Source: CAD feature listing. Evaluate the final solid. Frame: model axes, mm. Face numbers are marked on the shaded views. A direction names the side the tool comes from. Give positions to 0.01 mm unless a question says otherwise; leave off trailing zeros. Order: outer loops, then holes, each group sorted by start corner. A loop starts at its lowest first (then second) coordinate and runs counter-clockwise, first axis right, second up.
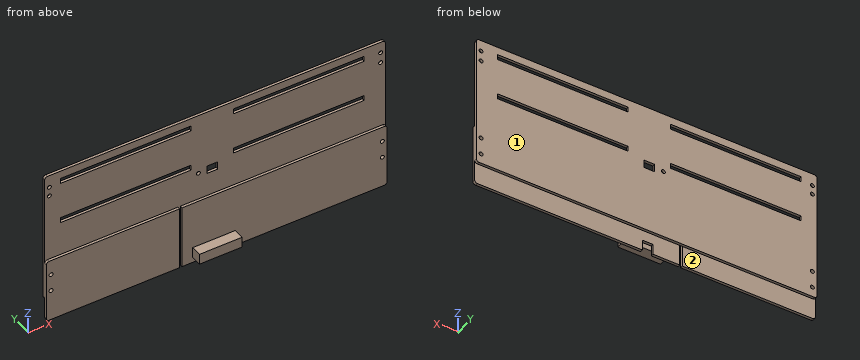
from build123d import *

# Parameters (mm, degrees)
F0_W      = 406.4
F0_H      = 158.75
F1_DEPTH  = 3.175
F2_R      = 3.175
F3_R      = 3.175
F4_R      = 3.175
F5_R      = 3.175
F6_W      = 155.575
F6_H      = 6.35
F7_DEPTH  = 3.175
F8_W      = 155.575
F8_H      = 6.35
F9_DEPTH  = 3.175
F10_W     = 155.575
F10_H     = 6.35
F11_DEPTH = 3.175
F12_W     = 155.575
F12_H     = 6.35
F13_DEPTH = 25.4
F14_W     = 12.7
F14_H     = 9.525
F15_DEPTH = 25.4
F16_R     = 2.38125
F17_DEPTH = 3.175
F18_R     = 2.38125
F19_DEPTH = 25.4
F20_R     = 2.38125
F21_DEPTH = 25.4
F22_W     = 406.4
F22_H     = 76.2
F23_DEPTH = 3.175
F24_R     = 3.175
F25_R     = 3.175
F26_W     = 12.7
F26_H     = 12.7
F27_DEPTH = 25.4
F28_R     = 2.38125
F29_DEPTH = 25.4
F30_W     = 50.8
F30_H     = 12.7
F31_DEPTH = 12.7
F32_W     = 3.175
F32_H     = 76.2
F33_DEPTH = 3.175


with BuildPart() as f1:
    # F0 (on Front) → F1 (new body)
    with BuildSketch(Plane.XZ):
        with Locations((8.5284784436, -21.1847552925)):
            Rectangle(F0_W, F0_H)
    extrude(amount=F1_DEPTH)

    # F2
    f2_edges = [f1.edges().sort_by_distance(p)[0] for p in [
        (-194.671522, -1.5875, 58.190245),
    ]]
    fillet(f2_edges, radius=F2_R)

    # F3
    f3_edges = [f1.edges().sort_by_distance(p)[0] for p in [
        (211.728478, -1.5875, 58.190245),
    ]]
    fillet(f3_edges, radius=F3_R)

    # F4
    f4_edges = [f1.edges().sort_by_distance(p)[0] for p in [
        (211.728478, -1.5875, -100.559755),
    ]]
    fillet(f4_edges, radius=F4_R)

    # F5
    f5_edges = [f1.edges().sort_by_distance(p)[0] for p in [
        (-194.671522, -1.5875, -100.559755),
    ]]
    fillet(f5_edges, radius=F5_R)

    # F6 (on face) → F7 (cut)
    with BuildSketch(Plane.XZ.offset(3.175)):
        with Locations((-97.8340215564, 45.4902447075)):
            Rectangle(F6_W, F6_H)
    extrude(amount=-F7_DEPTH, mode=Mode.SUBTRACT)

    # F8 (on face) → F9 (cut)
    with BuildSketch(Plane.XZ.offset(3.175)):
        with Locations((-97.8340215564, -5.3097552925)):
            Rectangle(F8_W, F8_H)
    extrude(amount=-F9_DEPTH, mode=Mode.SUBTRACT)

    # F10 (on face) → F11 (cut)
    with BuildSketch(Plane.XZ.offset(3.175)):
        with Locations((108.5409784436, 45.4902447075)):
            Rectangle(F10_W, F10_H)
    extrude(amount=-F11_DEPTH, mode=Mode.SUBTRACT)

    # F12 (on face) → F13 (cut)
    with BuildSketch(Plane.XZ.offset(3.175)):
        with Locations((108.5409784436, -5.3097552925)):
            Rectangle(F12_W, F12_H)
    extrude(amount=-F13_DEPTH, mode=Mode.SUBTRACT)

    # F14 (on face) → F15 (cut)
    with BuildSketch(Plane.XZ.offset(3.175)):
        with Locations((5.3534784436, -16.4222552925)):
            Rectangle(F14_W, F14_H)
    extrude(amount=-F15_DEPTH, mode=Mode.SUBTRACT)

    # F16 (on face) → F17 (cut)
    with BuildSketch(Plane.XZ.offset(3.175)):
        with Locations((-11.3152715564, -16.4666101336)):
            Circle(F16_R)
    extrude(amount=-F17_DEPTH, mode=Mode.SUBTRACT)

    # F18 (on face) → F19 (cut)
    with BuildSketch(Plane.XZ.offset(3.175)):
        with Locations((-189.1152715564, 43.1089947075)):
            Circle(F18_R)
        with Locations((-189.1152715564, 31.9964947075)):
            Circle(F18_R)
    extrude(amount=-F19_DEPTH, mode=Mode.SUBTRACT)

    # F20 (on face) → F21 (cut)
    with BuildSketch(Plane.XZ.offset(3.175)):
        with Locations((206.1722284436, 44.6964947075)):
            Circle(F20_R)
        with Locations((206.1722284436, 31.9964947075)):
            Circle(F20_R)
    extrude(amount=-F21_DEPTH, mode=Mode.SUBTRACT)

    # F22 (on face) → F23 (join)
    with BuildSketch(Plane.XZ.offset(3.175)):
        with Locations((8.5284784436, -87.8597552925)):
            Rectangle(F22_W, F22_H)
    extrude(amount=F23_DEPTH)

    # F24
    f24_edges = [f1.edges().sort_by_distance(p)[0] for p in [
        (-194.671522, -4.7625, -125.959755),
        (211.728478, -4.7625, -125.959755),
    ]]
    fillet(f24_edges, radius=F24_R)

    # F25
    f25_edges = [f1.edges().sort_by_distance(p)[0] for p in [
        (211.728478, -4.7625, -49.759755),
        (-194.671522, -4.7625, -49.759755),
    ]]
    fillet(f25_edges, radius=F25_R)

    # F26 (on face) → F27 (cut)
    with BuildSketch(Plane.XZ.offset(6.35)):
        with Locations((5.3534784436, -119.6097552925)):
            Rectangle(F26_W, F26_H)
    extrude(amount=-F27_DEPTH, mode=Mode.SUBTRACT)

    # F28 (on face) → F29 (cut)
    with BuildSketch(Plane.XZ.offset(6.35)):
        with Locations((206.1722284436, -68.0160052925)):
            Circle(F28_R)
        with Locations((206.1722284436, -88.6535052925)):
            Circle(F28_R)
        with Locations((-189.1152715564, -68.0160052925)):
            Circle(F28_R)
        with Locations((-189.1152715564, -88.6535052925)):
            Circle(F28_R)
    extrude(amount=-F29_DEPTH, mode=Mode.SUBTRACT)

    # F30 (on face) → F31 (join)
    with BuildSketch(Plane.XZ.offset(6.35)):
        with Locations((5.3534784436, -113.2597552925)):
            Rectangle(F30_W, F30_H)
    extrude(amount=F31_DEPTH)

    # F32 (on face) → F33 (cut)
    with BuildSketch(Plane.XZ.offset(6.35)):
        with Locations((-34.3340215564, -87.8597552925)):
            Rectangle(F32_W, F32_H)
    extrude(amount=-F33_DEPTH, mode=Mode.SUBTRACT)


solid = f1.part
1) Section query A-A on x = 150.5. Output: boundary loops of the cut face in (y, z) (3 decimals).
Checks:
outline: (-6.35, -125.96) - (-3.175, -125.96) - (-3.175, -100.56) - (0, -100.56) - (0, -8.485) - (-3.175, -8.485) - (-3.175, -49.76) - (-6.35, -49.76) - close; (-3.175, -2.135) - (0, -2.135) - (0, 42.315) - (-3.175, 42.315) - close; (-3.175, 48.665) - (0, 48.665) - (0, 58.19) - (-3.175, 58.19) - close
2) Section query B-B on y = -11.75. Output: boundary loops of the cut face in (x, z), and give its area (3 significant figures).
Checks:
outline: (-20.05, -119.61) - (30.75, -119.61) - (30.75, -106.91) - (-20.05, -106.91) - close
area: 645 mm2
3) Ray query, L1, parallel to Z at x = -120.5, y = -2.75; L2, parallel to X at y = -3.25, z = -63; L3, parallel to Z at x = 128.5, y = -6.25. Return the intervals inside material, ascending.
Checks:
L1: z = -100.56 to -8.48, -2.13 to 42.32, 48.67 to 58.19
L2: x = -194.67 to -35.92, -32.75 to 211.73
L3: z = -125.96 to -49.76
4) Reachability of the marked faces 1 and 2 from +Z, -Z, +X, -X, +Y, -Y: full face, straight path, thin tool, end or side. Return the list, or none.
Checks:
face 1: +Z, -Z, +X, -X, +Y
face 2: -Z, +X, -X, +Y
5) First-contact query: pin 1 Ø5 at (x, z) = (7, -116) entering from +Y; pin 2 Ø3.5 at (x, y) = (103, -5) entering from +Z; pin 3 Ø3.5 at (x, y) = (-78.5, -1) entering from -Z; pin 4 Ø4 at (y, z) = (-5.5, -29) entering from -X. Flat tips, straight axial feed; report the tip coordinate or a pass-through.
Checks:
pin 1: stops at y = -6.35
pin 2: stops at z = -49.76
pin 3: stops at z = -100.56
pin 4: passes through
6) Section query C-C on z = -35. Output: boundary loops of the cut face in (x, y) (3 decimals).
Checks:
outline: (-194.672, -3.175) - (211.728, -3.175) - (211.728, 0) - (-194.672, 0) - close
